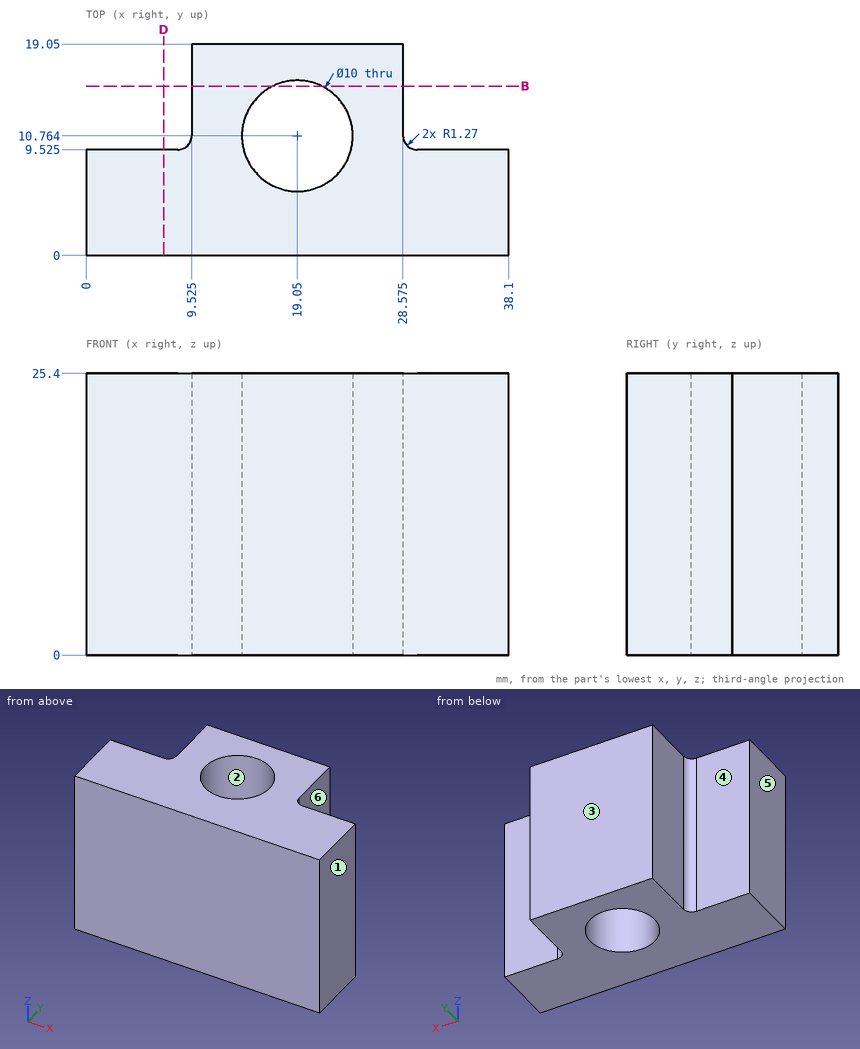
Study the drawing (mm; zero at the part's minimum x, y, z) and answer. A direction names the side the tool comes from. Coordinates: 2 decimals unless noted, no trailing zeros. Order: outer loops, then holes, each group sorted by start corner. A loop starts at its lowest first (then second) coordinate and runs counter-clockwise, first axis right, second up. Notation, with made-up numbers: M 88.25,-29.5 L 93.25,-29.5 A33 ccw 93.25,6.5 Z; hole C 76.5,-2.75 d9. An arc over 180 degrees is marked long. Answer as a JSON object with one key per item and string values. Group by question number.
1. Section D-D on x = 7 is taken. Write down the section's boundary in (y, z) (1 decimal).
2. A tool of negligible diameter and unlimited length cuts with its end or side. For the marked faces 4, 5 and 6, from which of +Z, -Z, +X, -X, +Y, -Y can it reach the whole face along a straight path? Write none if from no direction.
3. Flat-ended cylindrical pins translate along their axes: P1, Ø4, axis at y = 13, z = 17.5, coming from the -X side (1 decimal); P2, Ø4, axis at x = 32.5, z = 7, coming from the +Y side (1 decimal); P3, Ø6.5, axis at y = 15.5, z = 12.5, coming from the +X side (1 decimal). Find the tip coordinate at first contact, or state that the pin passes through.
4. Determine the mould class of the marked faces 1, 2 and 3 for opening direction X: released by +X, released by -X, zero draft, split by the parting line, or undercut.
5. Straight lines are drawn through the part: line 1 (Y direction, x = 33, z = 5.25) (1 decimal); line 2 (X direction, y = 13.25, z = 10.5) (1 decimal); line 3 (X direction, y = 17.5, z = 17) (1 decimal). For each, find the intervals that lie inside material, in ascending order.
6. Section B-B on y = 15.25 is taken. Write down the section's boundary in (x, z) (1 decimal).
Values follow:
{
 "1": {"outline": "M 0,0 L 9.5,0 L 9.5,25.4 L 0,25.4 Z"},
 "2": {"face 4": "+Z, -Z, -X, +Y", "face 5": "+Z, -Z, -X, +Y, -Y", "face 6": "+Z, -Z, +X, +Y"},
 "3": {"P1": "x = 9.5", "P2": "y = 9.5", "P3": "x = 28.6"},
 "4": {"face 1": "released by +X", "face 2": "undercut", "face 3": "zero draft"},
 "5": {"line 1": "0 to 9.5", "line 2": "9.5 to 14.7, 23.4 to 28.6", "line 3": "9.5 to 28.6"},
 "6": {"outline": "M 9.5,0 L 16.8,0 L 16.8,25.4 L 9.5,25.4 Z; M 21.3,0 L 28.6,0 L 28.6,25.4 L 21.3,25.4 Z"}
}
